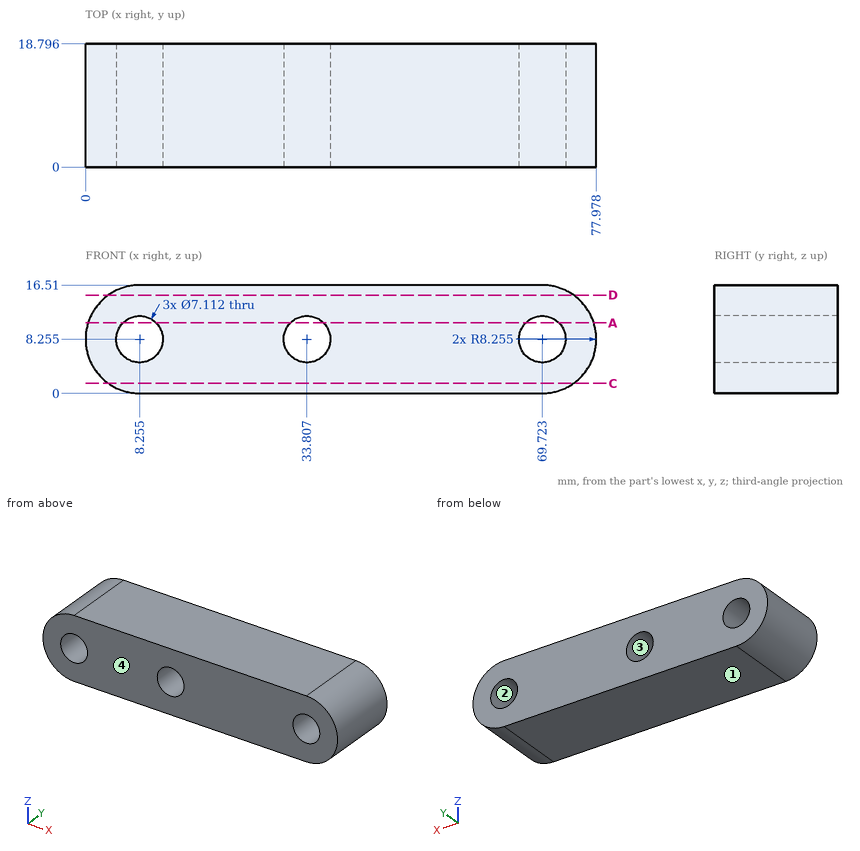
Here's the drawing with two shaded views (mm, measured from the low corner). I have some questions. Coordinates: 2 decimals unless noted, no trailing zeros. Write each loop counter-clockwise with the first axis right and the second up, starting at its lowest first coordinate (ties: lowest second). Pieces come first, ordered by that corner, then holes.
Item 1: If we mould it in two halves opening along Z, with no side actions, what happens to the marked faces 1, 2, 3 and 4? For each: +Z half, -Z half, draft (parallel to the pull), parting line (faces both ways), or undercut.
Item 2: I want a section at D-D on z = 15. Write out the boundary of the cut face in (x, y) (1 decimal), and give its area (3 significant figures).
Item 3: If I drill on line 1 (X direction, y = 3, z = 7.5) (1 decimal); line 2 (X direction, y = 3.75, z = 6.75) (1 decimal); line 3 (Z direction, x = 32, y = 16.25), over which ranges is the centre line in solid material (lowest first)?
Item 4: Will these pins go through, and if not, where does the flat tip stop? pin 1 (1.5 mm diameter, centred on y = 14.5, z = 11.5, fed in from -X); pin 2 (5 mm diameter, centred on y = 10, z = 2.5, fed in from -X); pin 3 (4 mm diameter, centred on y = 16, z = 11.5, fed in from +X).
Item 5: I want a section at C-C on z = 1.5. Write out the boundary of the cut face in (x, y).
Item 6: I want a section at A-A on z = 10.75. Write out the boundary of the cut face in (x, y), and give its area (3 significant figures).
Findings below:
1. face 1: -Z half
1. face 2: undercut
1. face 3: undercut
1. face 4: draft
2. outline: (3.5, 0) - (74.5, 0) - (74.5, 18.8) - (3.5, 18.8) - close
2. area: 1,330 mm2
3. line 1: x = 0 to 4.8, 11.7 to 30.3, 37.3 to 66.2, 73.2 to 77.9
3. line 2: x = 0.1 to 5, 11.5 to 30.6, 37 to 66.5, 72.9 to 77.8
3. line 3: z = 0 to 5.19, 11.32 to 16.51
4. pin 1: stops at x = 0.39
4. pin 2: stops at x = 0.67
4. pin 3: stops at x = 77.88
5. outline: (3.51, 0) - (74.47, 0) - (74.47, 18.8) - (3.51, 18.8) - close
6. outline: (0.39, 0) - (5.72, 0) - (5.72, 18.8) - (0.39, 18.8) - close; (10.79, 0) - (31.27, 0) - (31.27, 18.8) - (10.79, 18.8) - close; (36.34, 0) - (67.19, 0) - (67.19, 18.8) - (36.34, 18.8) - close; (72.26, 0) - (77.59, 0) - (77.59, 18.8) - (72.26, 18.8) - close
6. area: 1,170 mm2
